Source: CAD feature listing. Evaluate the final solid. Frame: model axes, mm. Face numbers are marked on the shaded views. A direction names the side the tool comes from. Round coordinates to 2 decimals unless told otherwise and drop trailing zeros. Order: outer loops, then holes, each group sorted by start corner. A loop starts at its lowest first (then second) coordinate and runs counter-clockwise, first axis right, second up. Notation, with made-up numbers: M 21,51.5 L 57,51.5 A11 cw 57,69.5 Z; hole C -34,-6.75 d10. An arc over 180 degrees is marked long. Use one line per item in the form item = value. Start each with the question number.
Q1. Section B-B (y = 2.25). Return the cut outline in (x, z), plus the area to 3 significant figures.
Q2. Pull-direction query (Z, two-part tool) for the marked faces 4, 5, 6 and 7; classes: pulls with the +Z half, pulls with the -Z half, needs draft (parallel to the pull), parting line crosses it, or undercut.
Q3. Section D-D (x = 20). Return the cut outline in (y, z) (1 decimal), plus the area to 3 significant figures.
Q4. Section A-A (x = 25.4). Return the cut outline in (y, z) (1 decimal), plus the area to 3 significant figures.
Q5. Contact query for flat-ended pins moving along their axis: pin 1 (4 mm diameter, centred on x = 6.35, z = -12.7, fed in from +Y); pin 2 (3 mm diameter, centred on x = 23.5, z = -17, fed in from -Y) (3 decimals); pin 3 (3 mm diameter, centred on y = 3.5, z = -8.5, fed in from +X) (3 decimals); pin 4 (7.5 mm diameter, centred on y = 3, z = -15.5, fed in from +X). Output: stop coordinate, or through.
Q6. Section C-C (z = -12.7). Return the cut outline in (x, y) (3 decimals).
Q7. Material intervals for probe 1 along Z at (x, y) = (25.4, 11.8); probe 2 along Z at (x, y) = (25.4, 6.5); probe 3 along Z at (x, y) = (6.35, 10.25), sorted ascending.
Q8. Reachability of the marked faces 1, 2 and 3 from +Z, -Z, +X, -X, +Y, -Y: full face, straight path, thin tool, end or side. Return the list, or none.
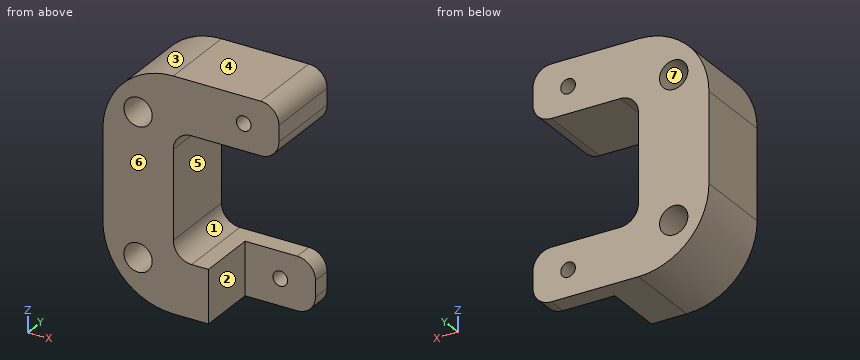
Autodesk Inventor part; units mm, degrees
ref_plane "YZ Plane" through (0, 0, 0) normal (1, 0, 0) x (0, 1, 0)
ref_plane "XZ Plane" through (0, 0, 0) normal (0, 1, 0) x (-1, 0, 0)
ref_plane "XY Plane" through (0, 0, 0) normal (0, 0, 1) x (1, 0, 0)
sketch "Sketch1" plane through (0, 0, 0) normal (1, 0, 0) x (0, 1, 0)
  line L0 (0, 20.7625) -> (0, -20.7625)
  line L1 (0, 20.7625) -> (14.224, 20.7625)
  line L2 (14.224, 20.7625) -> (14.224, 11.2375)
  line L3 (14.224, 11.2375) -> (6.35, 11.2375)
  line L4 (6.35, 11.2375) -> (6.35, -11.2375)
  line L5 (6.35, -11.2375) -> (14.224, -11.2375)
  line L6 (14.224, -11.2375) -> (14.224, -20.7625)
  line L7 (14.224, -20.7625) -> (0, -20.7625)
  point P0 (0, 0)
  point P1 (0, 0)
  point P2 (14.224, -16)
  point P3 (14.224, 16)
  dimension "d1" = 32
  dimension "d2" = 7.874
  dimension "d4" = 6.35
  dimension "d5" = 9.525
extrude "Extrusion1" add sketch "Sketch1" along normal blind 31.75
sketch "Sketch2" plane through (0, 14.224, 20.7625) normal (0, 1, 0) x (1, 0, 0)
  line L0 (0, 9.525) -> (31.75, 9.525) construction
  line L1 (31.75, 9.525) -> (31.75, 0) construction
  line L2 (31.75, 0) -> (0, 0) construction
  line L3 (0, 0) -> (0, 9.525) construction
  line L4 (0, 41.525) -> (31.75, 41.525) construction
  line L5 (31.75, 41.525) -> (31.75, 32) construction
  line L6 (31.75, 32) -> (0, 32) construction
  line L7 (0, 32) -> (0, 41.525) construction
  point P0 (0, 20.7625)
  point P1 (25.4, 4.7625)
  point P2 (25.4, 36.7625)
  point P3 (31.75, 4.7625)
  point P4 (31.75, 36.7625)
  dimension "d8" = 6.35
hole "Hole1" at (25.4, 14.224, 16) at (25.4, 14.224, -16) direction (0, -1, 0) diameter 2.6416 end through all
sketch "Sketch4" plane through (0, 6.35, 11.2375) normal (0, 1, 0) x (1, 0, 0)
  circle A0 centre (25.4, -4.7625) radius 1.3208 construction
  circle A1 centre (25.4, 27.2375) radius 1.3208 construction
  line L0 (0, 32) -> (31.75, 32) construction
  line L1 (31.75, 32) -> (31.75, 22.475) construction
  line L2 (31.75, 22.475) -> (0, 22.475) construction
  line L3 (0, 0) -> (0, 22.475) construction
  line L4 (0, 0) -> (31.75, 0) construction
  line L5 (31.75, 0) -> (31.75, -9.525) construction
  line L6 (31.75, -9.525) -> (0, -9.525) construction
  line L7 (0, -9.525) -> (0, 0) construction
  line L8 (0, 22.475) -> (0, 32) construction
  line L9 (31.75, 22.475) -> (31.75, 0) construction
  line L10 (0, 22.475) -> (31.75, 22.475) construction
  line L11 (31.75, 0) -> (12.7, 0)
  line L12 (12.7, 0) -> (12.7, 22.475)
  line L13 (12.7, 22.475) -> (31.75, 22.475)
  line L14 (31.75, 22.475) -> (31.75, 0)
  point P0 (0, 11.2375)
  point P1 (14.7922, 22.475)
  dimension "d25" = 19.05
extrude "Extrusion2" cut sketch "Sketch4" along normal mid plane 38.1
sketch "Sketch5" plane through (0, 14.224, 20.7625) normal (0, 1, 0) x (1, 0, 0)
  line L0 (0, 0) -> (0, 41.525) construction
  line L1 (0, 41.525) -> (31.75, 41.525) construction
  line L2 (0, 41.525) -> (12.7, 41.525)
  line L3 (12.7, 41.525) -> (12.7, 0.1925)
  line L4 (12.7, 0.1925) -> (0, 0.1925)
  line L5 (0, 0.1925) -> (0, 41.525)
  line L6 (12.7, 9.525) -> (12.7, 32) construction
  point P0 (0, 20.7625)
extrude "Extrusion3" add sketch "Sketch5" against normal up to surface (7.874 mm away)
sketch "Sketch6" plane through (0, 14.224, 20.7625) normal (0, 1, 0) x (1, 0, 0)
  line L0 (6.35, 8.0625) -> (6.35, 33.4625) construction
  line L1 (0, 41.525) -> (0, 0) construction
  point P0 (0, 20.7625)
  point P1 (6.35, 20.7625)
  point P2 (0, 20.7625)
  dimension "d30" = 6.35
  dimension "d31" = 25.4
hole "Hole3" at (6.35, 14.224, 12.7) at (6.35, 14.224, -12.7) direction (0, -1, 0) diameter 5.1054 end through all
fillet "Fillet1" radius 12.7 2 edges at (0, 7.112, -20.7625) (0, 7.112, 20.7625)
fillet "Fillet2" radius 3.302 6 edges at (12.7, 7.112, -11.2375) (12.7, 7.112, 11.2375) (31.75, 7.112, 20.7625) (31.75, 7.112, 11.2375) (31.75, 7.112, -11.2375) (31.75, 7.112, -20.7625)
sketch "Sketch7" plane through (0, 0, -8.0625) normal (0, -1, 0) x (1, 0, 0)
  arc A0 (16.002, 19.3) -> (12.7, 15.998) centre (16.002, 15.998) ccw construction
  line L0 (12.7, 15.998) -> (12.7, 0.127) construction
  arc A1 (12.7, 0.127) -> (16.002, -3.175) centre (16.002, 0.127) ccw construction
  line L1 (16.002, -3.175) -> (28.448, -3.175) construction
  arc A2 (31.75, -6.477) -> (28.448, -3.175) centre (28.448, -6.477) ccw
  line L2 (31.75, -6.477) -> (31.75, -9.398)
  arc A3 (28.448, -12.7) -> (31.75, -9.398) centre (28.448, -9.398) ccw
  line L3 (28.448, -12.7) -> (12.7, -12.7) construction
  arc A4 (0, 0) -> (12.7, -12.7) centre (12.7, 0) ccw construction
  line L4 (0, 0) -> (0, 16.125) construction
  arc A5 (12.7, 28.825) -> (0, 16.125) centre (12.7, 16.125) ccw construction
  line L5 (12.7, 28.825) -> (28.448, 28.825) construction
  arc A6 (31.75, 25.523) -> (28.448, 28.825) centre (28.448, 25.523) ccw construction
  line L6 (31.75, 25.523) -> (31.75, 22.602) construction
  arc A7 (28.448, 19.3) -> (31.75, 22.602) centre (28.448, 22.602) ccw construction
  line L7 (28.448, 19.3) -> (16.002, 19.3) construction
  circle A8 centre (6.35, 20.7625) radius 2.5527 construction
  circle A9 centre (6.35, -4.6375) radius 2.5527 construction
  circle A10 centre (25.4, 24.0625) radius 1.3208 construction
  circle A11 centre (25.4, -7.9375) radius 1.3208
  line L8 (12.7, -12.7) -> (28.448, -12.7) construction
  line L9 (28.448, -12.7) -> (19.05, -12.7)
  line L10 (19.05, -12.7) -> (19.05, -3.175)
  line L11 (16.002, -3.175) -> (28.448, -3.175) construction
  line L12 (19.05, -3.175) -> (28.448, -3.175)
  point P0 (0, 8.0625)
  dimension "d41" = 12.7
extrude "Extrusion4" cut sketch "Sketch7" against normal blind 10.795
properties part number "GP7-006" material "Aluminum 6061"
Results list:
q1.outline = M 0,-8.06 A12.7 ccw 12.7,-20.76 L 19.05,-20.76 L 19.05,-11.24 L 16,-11.24 A3.3 cw 12.7,-7.94 L 12.7,7.94 A3.3 cw 16,11.24 L 28.45,11.24 A3.3 ccw 31.75,14.54 L 31.75,17.46 A3.3 ccw 28.45,20.76 L 12.7,20.76 A12.7 ccw 0,8.06 Z; hole C 6.35,-12.7 d5.11; hole C 6.35,12.7 d5.11; hole C 25.4,16 d2.64
q1.area = 654 mm2
q2.face_4 = pulls with the +Z half
q2.face_5 = undercut
q2.face_6 = needs draft
q2.face_7 = undercut
q3.outline = M 0,11.2 L 14.2,11.2 L 14.2,20.8 L 0,20.8 Z; M 10.8,-20.8 L 14.2,-20.8 L 14.2,-11.2 L 10.8,-11.2 Z
q3.area = 168 mm2
q4.outline = M 0,11.2 L 14.2,11.2 L 14.2,14.7 L 0,14.7 Z; M 0,17.3 L 14.2,17.3 L 14.2,20.8 L 0,20.8 Z; M 10.8,-20.8 L 14.2,-20.8 L 14.2,-17.3 L 10.8,-17.3 Z; M 10.8,-14.7 L 14.2,-14.7 L 14.2,-11.2 L 10.8,-11.2 Z
q4.area = 122 mm2
q5.pin_1 = through
q5.pin_2 = 10.795
q5.pin_3 = 13.425
q5.pin_4 = 19.05
q6.outline = M 0.877,0 L 3.797,0 L 3.797,14.224 L 0.877,14.224 Z; M 8.903,0 L 19.05,0 L 19.05,10.795 L 31.19,10.795 L 31.19,14.224 L 8.903,14.224 Z
q7.probe_1 = -20.76 to -17.32, -14.68 to -11.24, 11.24 to 14.68, 17.32 to 20.76
q7.probe_2 = 11.24 to 14.68, 17.32 to 20.76
q7.probe_3 = -19.06 to -15.25, -10.15 to 10.15, 15.25 to 19.06
q8.face_1 = +X, +Y, -Y
q8.face_2 = -Z, +X, -Y
q8.face_3 = +Z, -X, +Y, -Y
